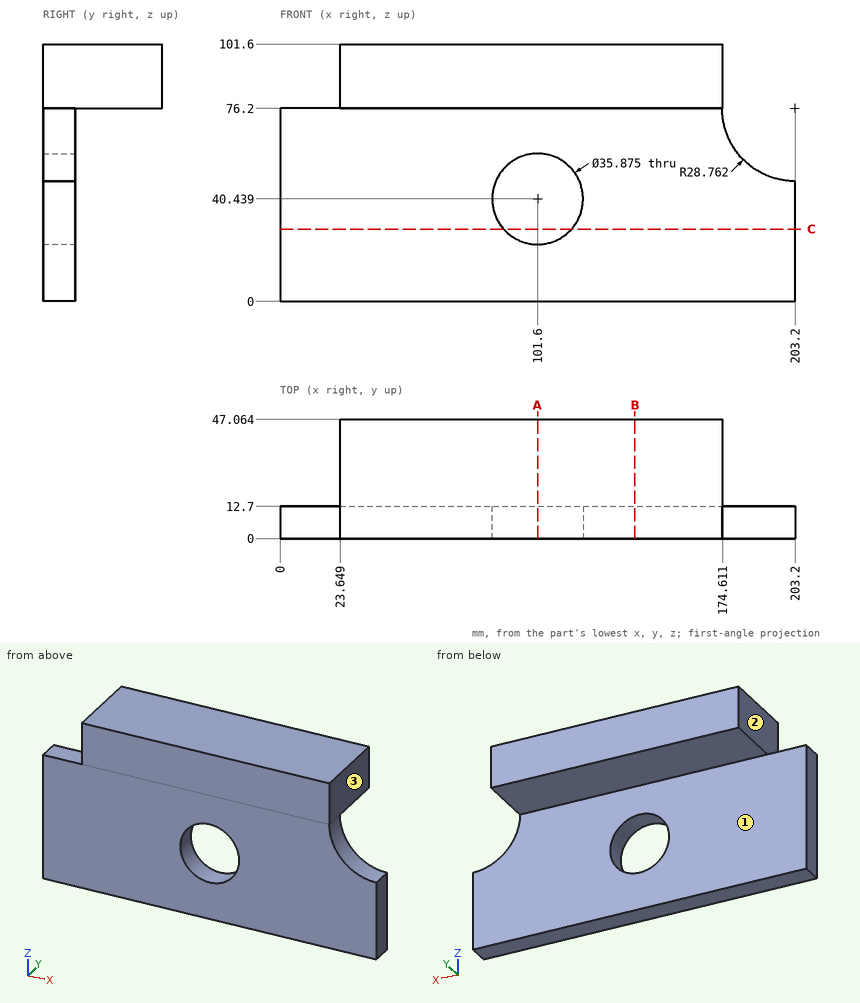
Answer from the drawing. Dimensions are ordinates in mm from the lowest x, y and z of the part. A direction names the side the tool comes from. Round coordinates to 2 decimals unless told otherwise and drop trailing zeros. Order: outer loops, then holes, each group sorted by start corner. A loop starts at its lowest first (then second) coordinate and runs counter-clockwise, first axis right, second up. Notation, with made-up numbers: (30, 39.5) - (68, 39.5) arc R15 ccw to (68, 43.5) - close; hole circle Ø4 at (19, 55.25). An arc over 180 degrees is marked (long way). Put each result on its own line as item: value. Start each with the question number.
(1) Straight lines are drawn through the part: probe 1 along Z at (x, y) = (101.6, 7.5); probe 2 along Z at (x, y) = (57.5, 31); probe 3 along Y at (x, z) = (157.5, 26). For each, find the intervals that lie inside material, in ascending order. Write a range as from..to.
(2) Find section A-A (x = 101.6). Give the vertices of the cut face in (y, z).
(3) For the marked faces 1, 2 and 3, determine the directions among +Z, -Z, +X, -X, +Y, -Y from which every point of the face is accessible in a straight line to the end or side of a thin tool.
(4) Given P1, Ø1, axis at x = 52.5, z = 69, coming from the +Y side; P2, Ø12.5, axis at y = 12, z = 92, coming from the -X side; P3, Ø12.5, axis at y = 30.5, z = 83, coming from the +X side, each flat-ended and moving along its own axis, determine where each tip first touches the part or whether it passes through.
(5) Find section B-B (x = 140). Give the vertices of the cut face in (y, z).
(6) Find section C-C (z = 28.5). Give the vertices of the cut face in (x, y), plus the area to 3 significant figures.
Reply:
1. probe 1: 0..22.5, 58.38..101.6
1. probe 2: 76.2..101.6
1. probe 3: 0..12.7
2. outline: (0, 0) - (12.7, 0) - (12.7, 22.5) - (0, 22.5) - close; (0, 58.38) - (12.7, 58.38) - (12.7, 76.2) - (47.06, 76.2) - (47.06, 101.6) - (0, 101.6) - close
3. face 1: -Z, +X, -X, +Y
3. face 2: +Z, -X, +Y, -Y
3. face 3: +Z, +X, +Y, -Y
4. P1: y = 12.7
4. P2: x = 23.65
4. P3: x = 174.61
5. outline: (0, 0) - (12.7, 0) - (12.7, 76.2) - (47.06, 76.2) - (47.06, 101.6) - (0, 101.6) - close
6. outline: (0, 0) - (88.21, 0) - (88.21, 12.7) - (0, 12.7) - close; (114.99, 0) - (203.2, 0) - (203.2, 12.7) - (114.99, 12.7) - close
6. area: 2,240 mm^2
